Could you check a few things on this drawing? It's one solid part, dimensions in mm from its lowest x, y, z. A direction names the side the tool comes from. Give positions to 0.01 mm unless a question says otherwise; leave off trailing zeros. Order: outer loops, then holes, each group sorted by start corner. A loop starts at its lowest first (then second) coordinate and runs counter-clockwise, first axis right, second up.
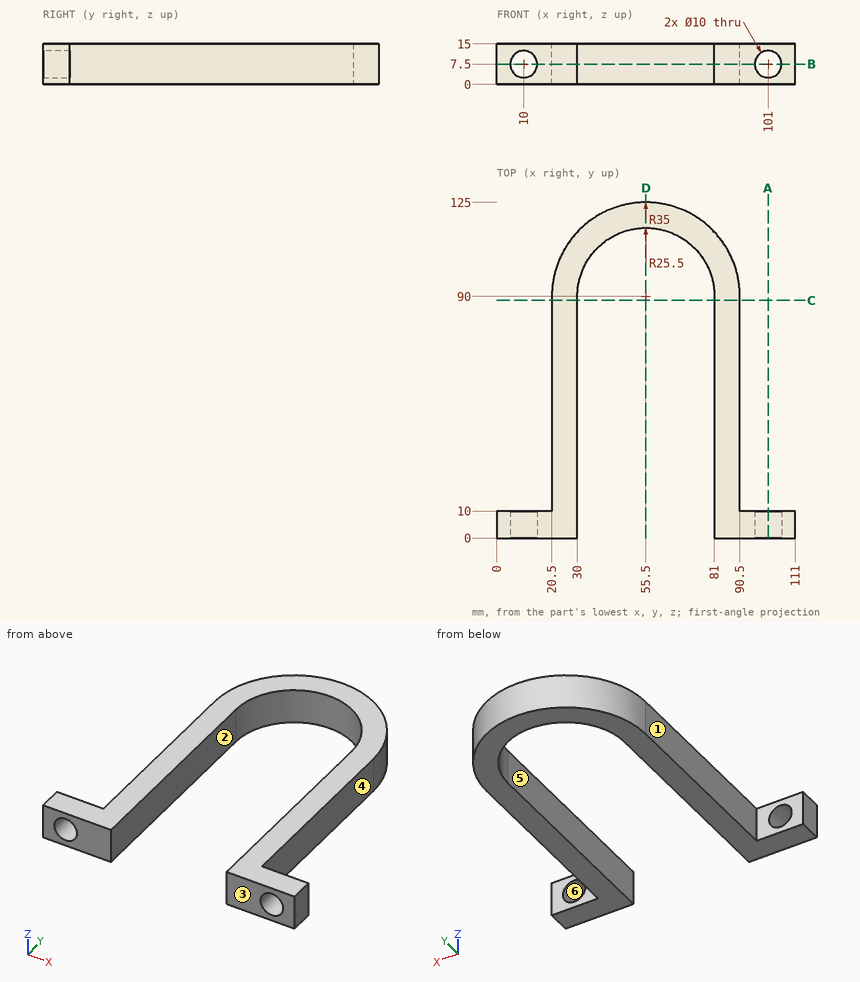
1) Suppose I cut it at A-A (x = 101). Please give me the cut outline in (y, z).
2) Suppose I cut it at B-B (z = 7.5). Please give me the cut outline in (x, y).
3) Suppose I cut it at C-C (y = 88.5). Please give me the cut outline in (x, z), and give its area (3 significant figures).
4) If I drill on line 1 (X direction, y = 5, z = 7.5); line 2 (X direction, y = 52.5, z = 7); line 3 (Y direction, x = 20, z = 13.25), over which ranges is the centre line in solid material (lowest first)?
5) Suppose I cut it at D-D (x = 55.5). Please give me the cut outline in (y, z).
6) We'd pull the mould along X, two halves only. Please class the marked faces 1, 2 and 3: +X half, -X half, draft (parallel to the pull), parting line (faces both ways), or undercut.
7) Which directions (+Z, -Z, +X, -X, +Y, -Y) give clear straight access to the entire face, cutting with the end or side of a thin tool? Please do the marked faces 4, 5 and 6.
8) I'm going to push flat-ended pins straight in: pin 1 Ø1 at (y, z) = (99.5, 9.5) entering from -X; pin 2 Ø7.5 at (y, z) = (30.5, 6) entering from +X; pin 3 Ø7.5 at (y, z) = (65.5, 8.5) entering from -X; pin 4 Ø8 at (x, z) = (101, 7.5) entering from +Y. Where does each tip first touch, or does it pass through?
Results:
1. outline: (0, 0) - (10, 0) - (10, 2.5) - (0, 2.5) - close; (0, 12.5) - (10, 12.5) - (10, 15) - (0, 15) - close
2. outline: (0, 0) - (5, 0) - (5, 10) - (0, 10) - close; (15, 0) - (30, 0) - (30, 90) arc R25.5 cw to (81, 90) - (81, 0) - (96, 0) - (96, 10) - (90.5, 10) - (90.5, 90) arc R35 ccw to (20.5, 90) - (20.5, 10) - (15, 10) - close; (106, 0) - (111, 0) - (111, 10) - (106, 10) - close
3. outline: (20.5, 0) - (30, 0) - (30, 15) - (20.5, 15) - close; (81, 0) - (90.5, 0) - (90.5, 15) - (81, 15) - close
3. area: 285 mm2
4. line 1: x = 0 to 5, 15 to 30, 81 to 96, 106 to 111
4. line 2: x = 20.5 to 30, 81 to 90.5
4. line 3: y = 0 to 10
5. outline: (115.5, 0) - (125, 0) - (125, 15) - (115.5, 15) - close
6. face 1: -X half
6. face 2: undercut
6. face 3: draft
7. face 4: +Z, -Z, +X, +Y
7. face 5: +Z, -Z, -Y
7. face 6: +Y, -Y
8. pin 1: stops at x = 21.68
8. pin 2: stops at x = 90.5
8. pin 3: stops at x = 20.5
8. pin 4: passes through
